Can you work these out from the model? Positions are in its coordinate system, mm. A direction names the side the tool comes from. Round coordinates to 2 decimals unless told otherwise and drop trailing zeros. Loops run counter-clockwise (first coordinate to the right, second up) from the corner with the lowest first, then second, coordinate; pieces in that order, holes last. Notation, with made-up numbers: (-15.5, 77.5) -> (29.5, 77.5) arc R27 ccw to (29.5, 107.5) -> close; hole circle Ø11 at (-25.5, -24.5). An arc over 180 degrees is marked (long way). Write each question's results on one line, items separated by ' | '.
from build123d import *

# Parameters (mm, degrees)
F0_W     = 127
F0_H     = 127
F0_R     = 6.35
F1_DEPTH = 6.35
F2_W     = 76.2
F2_H     = 76.2
F2_R     = 15.875
F3_DEPTH = 127


with BuildPart() as f1:
    # F0 (on Top) → F1 (new body)
    with BuildSketch(Plane.XY):
        Rectangle(F0_W, F0_H)
        with Locations((-50.8, -50.8)):
            Circle(F0_R, mode=Mode.SUBTRACT)
        with Locations((50.8, -50.8)):
            Circle(F0_R, mode=Mode.SUBTRACT)
        with Locations((-50.8, 50.8)):
            Circle(F0_R, mode=Mode.SUBTRACT)
        with Locations((50.8, 50.8)):
            Circle(F0_R, mode=Mode.SUBTRACT)
    extrude(amount=F1_DEPTH)

    # F2 (on face) → F3 (join, through all)
    with BuildSketch(Plane.XZ.offset(63.5)):
        with Locations((0, 44.45)):
            Rectangle(F2_W, F2_H)
        with Locations((0, 50.8)):
            Circle(F2_R, mode=Mode.SUBTRACT)
    extrude(amount=-F3_DEPTH)


solid = f1.part
1. If we section it at D-D (y = 10): List the corners of the cut face in (x, z) for me (3 decimals).
Final values:
outline: (-63.5, 0) -> (63.5, 0) -> (63.5, 6.35) -> (38.1, 6.35) -> (38.1, 82.55) -> (-38.1, 82.55) -> (-38.1, 6.35) -> (-63.5, 6.35) -> close; hole circle Ø31.75 at (0, 50.8)
2. If we section it at B-B (y = 50.8): List the corners of the cut face in (x, z) for me (3 decimals), then the cut area to 3 significant figures.
Final values:
outline: (-63.5, 0) -> (-57.15, 0) -> (-57.15, 6.35) -> (-63.5, 6.35) -> close; (-44.45, 0) -> (44.45, 0) -> (44.45, 6.35) -> (38.1, 6.35) -> (38.1, 82.55) -> (-38.1, 82.55) -> (-38.1, 6.35) -> (-44.45, 6.35) -> close; (57.15, 0) -> (63.5, 0) -> (63.5, 6.35) -> (57.15, 6.35) -> close; hole circle Ø31.75 at (0, 50.8) | area: 5,660 mm2
3. If we section it at C-C (z = 50.8): List the corners of the cut face in (x, y) for me (3 decimals), then the cut area to 3 significant figures.
Final values:
outline: (-38.1, -63.5) -> (-15.875, -63.5) -> (-15.875, 63.5) -> (-38.1, 63.5) -> close; (15.875, -63.5) -> (38.1, -63.5) -> (38.1, 63.5) -> (15.875, 63.5) -> close | area: 5,650 mm2
4. We'd pull the mould along X, two halves only. Please class faces 1 (the face through (-44.743, -48.893, 3.131)), 2 (the face through (38.1, -1, 44)), 3 (the face through (-63.5, -1, 3)), 4 (the face through (-51, 1, 6.35)): pulls with the +X half, pulls with the -X half, needs draft (parallel to the pull), parting line crosses it, or undercut.
Final values:
face 1: undercut | face 2: pulls with the +X half | face 3: pulls with the -X half | face 4: needs draft
5. Please list where these lines run through material, in increasing order: line 1 (Y direction, x = -50.8, z = 3.75); line 2 (X direction, y = -50, z = 1); line 3 (Z direction, x = 0, y = 17) (3 decimals). Write a range as from..to.
Final values:
line 1: -63.5..-57.15, -44.45..44.45, 57.15..63.5 | line 2: -63.5..-57.1, -44.5..44.5, 57.1..63.5 | line 3: 0..34.925, 66.675..82.55
6. Will these pins go through, and if not, where does the flat tip stop? pin 1 (20.5 mm diameter, centred on x = 56.5, y = -13.5, fed in from +Z); pin 2 (6 mm diameter, centred on y = 27.5, z = 25.5, fed in from -X); pin 3 (7.5 mm diameter, centred on x = -47, y = -13.5, fed in from +Z).
Final values:
pin 1: z = 6.35 | pin 2: x = -38.1 | pin 3: z = 6.35
7. If we section it at A-A (x = 0): List the corners of the cut face in (y, z) for me (3 decimals).
Final values:
outline: (-63.5, 0) -> (63.5, 0) -> (63.5, 34.925) -> (-63.5, 34.925) -> close; (-63.5, 66.675) -> (63.5, 66.675) -> (63.5, 82.55) -> (-63.5, 82.55) -> close
8. On a 3-axis mill with a long thin cutter (end or side, diameter ignored), from which of +Z, -Z, +X, -X, +Y, -Y can I reach the whole of each face in a straight line? I mean faces 5 (the face through (56.857, 52.707, 3.131)), 6 (the face through (-38.1, -1, 44)), 7 (the face through (51, 1, 6.35)). Say none if no direction works.
Final values:
face 5: +Z, -Z | face 6: +Z, -X, +Y, -Y | face 7: +Z, +X, +Y, -Y
